Geometry check sheet. Reference: drawing and pictorial views, mm from the part's lowest x, y, z. Give positions to 0.01 mm unless a question says otherwise; leave off trailing zeros. Loops run counter-clockwise (first coordinate to the right, second up) from the corner with the lowest first, then second, coordinate; pieces in that order, holes last. Notation, with made-up numbers: (-14, 68.5) -> (40, 68.5) arc R25 cw to (40, 92.5) -> close; hole circle Ø5 at (67.5, -0.75). An arc over 180 degrees is marked (long way). Write item = value, one per line. Start each with the question number.
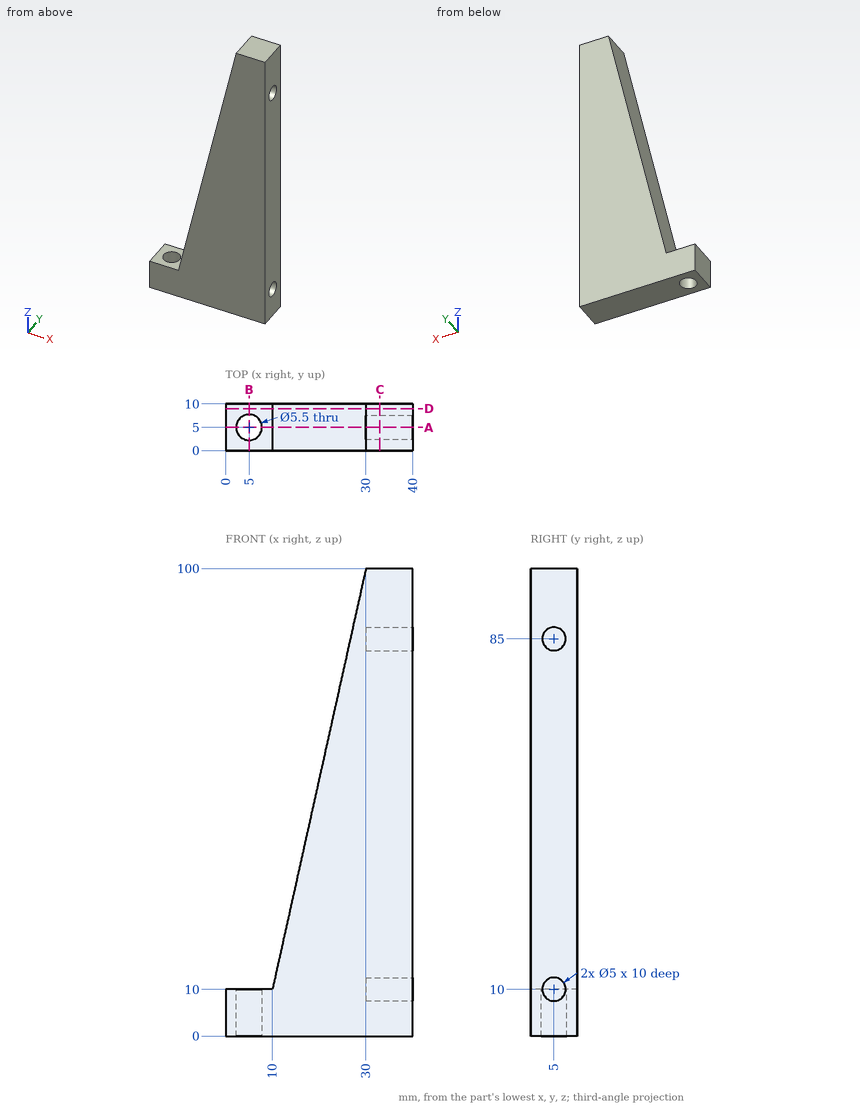
1) Thickness scan on line 1 (Z direction, x = 35, y = 5); line 2 (Y direction, x = 5, z = 6); line 3 (Z direction, x = 8.5, y = 8.5). Record the ranges inside material, lowest first.
2) Section check D-D (y = 9). Enter the section's corners in (x, z).
3) Depth check by flat-ended pin: pin 1 Ø3 at (x, y) = (4.5, 7) entering from +Z; pin 2 Ø6 at (y, z) = (2, 17) entering from -X; pin 3 Ø1.5 at (y, z) = (4, 9.5) entering from +X. Enter the tip coordinate at first touch or a pass-through.
4) Section check B-B (x = 5). Enter the section's corners in (y, z).
5) Section check A-A (y = 5). Enter the section's corners in (x, z).
6) Section check C-C (x = 33). Enter the section's corners in (y, z), plus the area to 3 significant figures.
Check result:
q1.line_1 = 0 to 7.5, 12.5 to 82.5, 87.5 to 100
q1.line_2 = 0 to 2.25, 7.75 to 10
q1.line_3 = 0 to 10
q2.outline = (0, 0) -> (40, 0) -> (40, 100) -> (30, 100) -> (10, 10) -> (0, 10) -> close
q3.pin_1 = 10
q3.pin_2 = 10.89
q3.pin_3 = 30
q4.outline = (0, 0) -> (2.25, 0) -> (2.25, 10) -> (0, 10) -> close; (7.75, 0) -> (10, 0) -> (10, 10) -> (7.75, 10) -> close
q5.outline = (0, 0) -> (2.25, 0) -> (2.25, 10) -> (0, 10) -> close; (7.75, 0) -> (40, 0) -> (40, 7.5) -> (30, 7.5) -> (30, 12.5) -> (40, 12.5) -> (40, 82.5) -> (30, 82.5) -> (30, 87.5) -> (40, 87.5) -> (40, 100) -> (30, 100) -> (10, 10) -> (7.75, 10) -> close
q6.outline = (0, 0) -> (10, 0) -> (10, 100) -> (0, 100) -> close; hole circle Ø5 at (5, 10); hole circle Ø5 at (5, 85)
q6.area = 961 mm2
